Study the drawing (mm; zero at the part's minimum x, y, z) and answer. Coordinates: 2 decimals unless noted, no trailing zeros. Write each loop counter-clockwise with the first axis right and the second up, starting at its lowest first coordinate (ties: lowest second). Pieces come first, ordered by that corner, then holes. Notation, with made-up numbers: (12, 16) -> (40, 16) arc R26 cw to (40, 34) -> close; hole circle Ø4 at (-32.5, -34.75). An arc over 180 degrees is marked (long way). Answer in a Markdown table with one row per item. Add a question column.
Item 1: Section A-A on x = 80 is taken. Write down the section's boundary in (y, z) (3 decimals).
Item 2: Section B-B on y = 35 is taken. Write down the section's boundary in (x, z) (3 decimals).
Item 3: Straight lines are drawn through the part: line 1 (Y direction, x = 6, z = 1.5); line 2 (X direction, y = 39.5, z = 2.9); line 3 (X direction, y = 11.5, z = 1.6). For each, find the intervals that lie inside material, in ascending order. Write a range as from..to.
Item 4: Given pin 1 Ø1 at (x, z) = (23.5, 2) entering from +Y, flat-ended and moving along its own axis, determine where the tip first touches the part or whether it passes through.
Item 5: Section D-D on x = 33.5 is taken. Write down the section's boundary in (y, z) (3 decimals).
Item 6: Section C-C on y = 15 is taken. Write down the section's boundary in (x, z) (3 decimals), then the cut area to 3 significant figures.
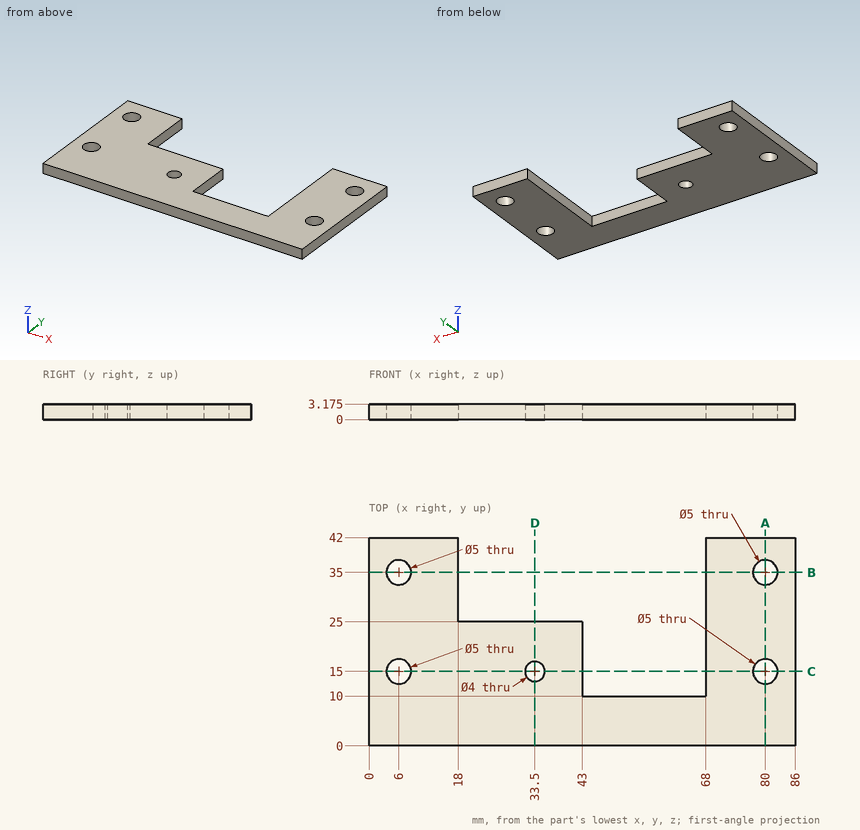
Results below:
| question | item | result |
|---|---|---|
| 1 | outline | (0, 0) -> (12.5, 0) -> (12.5, 3.175) -> (0, 3.175) -> close; (17.5, 0) -> (32.5, 0) -> (32.5, 3.175) -> (17.5, 3.175) -> close; (37.5, 0) -> (42, 0) -> (42, 3.175) -> (37.5, 3.175) -> close |
| 2 | outline | (0, 0) -> (3.5, 0) -> (3.5, 3.175) -> (0, 3.175) -> close; (8.5, 0) -> (18, 0) -> (18, 3.175) -> (8.5, 3.175) -> close; (68, 0) -> (77.5, 0) -> (77.5, 3.175) -> (68, 3.175) -> close; (82.5, 0) -> (86, 0) -> (86, 3.175) -> (82.5, 3.175) -> close |
| 3 | line 1 | y = 0..12.5, 17.5..32.5, 37.5..42 |
| 3 | line 2 | x = 0..18, 68..86 |
| 3 | line 3 | x = 0..43, 68..86 |
| 4 | pin 1 | stops at y = 25 |
| 5 | outline | (0, 0) -> (13, 0) -> (13, 3.175) -> (0, 3.175) -> close; (17, 0) -> (25, 0) -> (25, 3.175) -> (17, 3.175) -> close |
| 6 | outline | (0, 0) -> (3.5, 0) -> (3.5, 3.175) -> (0, 3.175) -> close; (8.5, 0) -> (31.5, 0) -> (31.5, 3.175) -> (8.5, 3.175) -> close; (35.5, 0) -> (43, 0) -> (43, 3.175) -> (35.5, 3.175) -> close; (68, 0) -> (77.5, 0) -> (77.5, 3.175) -> (68, 3.175) -> close; (82.5, 0) -> (86, 0) -> (86, 3.175) -> (82.5, 3.175) -> close |
| 6 | area | 149 mm2 |
